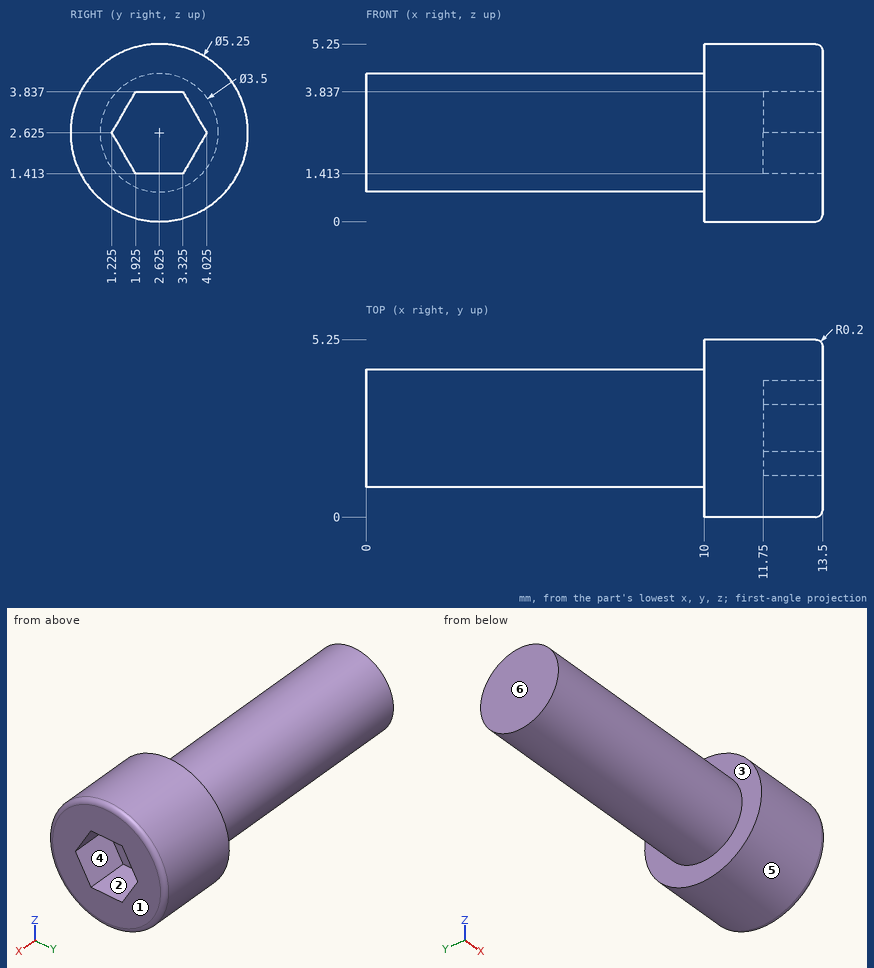
Here's the drawing with two shaded views (mm, measured from the low corner). I have some questions. A direction names the side the tool comes from. Round coordinates to 2 decimals unless told otherwise and drop trailing zeros. Write each question's results on one line, items separated by ' | '. Start each with the question number.
Item 1: Will these pins go through, and if not, where does the flat tip stop? pin 1 (1.9 mm diameter, centred on y = 2, z = 2, fed in from +X); pin 2 (1 mm diameter, centred on x = 7, z = 4.5, fed in from -Y); pin 3 (1 mm diameter, centred on x = 1.5, y = 1, fed in from +Z) (1 decimal).
Item 2: Thinking about a two-plate mould opening in Z: for the marked faces 4, 5 and 6, which applies, +Z half, -Z half, draft (parallel to the pull), parting line (faces both ways), or undercut?
Item 3: Please list where these lines run through material, in increasing order: L1, parallel to X at y = 2.2, z = 3.05; L2, parallel to X at y = 3.2, z = 4.6; L3, parallel to Z at x = 8.5, y = 2.55.
Item 4: Which directions (+Z, -Z, +X, -X, +Y, -Y) give clear straight access to the entire face, cutting with the end or side of a thin tool? Please do the marked faces 1, 2 and 3.
Results:
1) pin 1: stops at x = 13.5 | pin 2: stops at y = 1.54 | pin 3: stops at z = 4
2) face 4: undercut | face 5: parting line | face 6: draft
3) L1: x = 0 to 11.75 | L2: x = 10 to 13.5 | L3: z = 0.88 to 4.37
4) face 1: +Z, -Z, +X, +Y, -Y | face 2: +X | face 3: -X
